Job drawing, mm, ordinate dimensions from the low corner. One solid piece. Round coordinates to 2 decimals unless told otherwise and drop trailing zeros. Loops run counter-clockwise (first coordinate to the right, second up) from the corner with the lowest first, then second, coordinate; pieces in that order, holes last.
1) Band-saw the part on D-D, the plane x = 29. Write the cut outline in (y, z) (1 decimal), then the cut area to 3 significant figures.
2) Band-saw the part on B-B, the plane x = 19.8. Write the cut outline in (y, z) (1 decimal).
3) Mould opens along Z. For the marked faces 1, 2, 3 and 4 say: +Z half, -Z half, draft (parallel to the pull), parting line (faces both ways), or undercut.
4) Drop flat-ended pins along their axis: P1, Ø2, axis at y = 1, z = 47, coming from the -X side; P2, Ø8, axis at y = 28.5, z = 35.5, coming from the +X side; P3, Ø19, axis at x = 20, y = 12.5, coming from the +Z side (1 decimal). Give the stop position or say it passes through.
5) Band-saw the part on C-C, the plane y = 15. Write the cut outline in (x, z) (1 decimal).
6) Probe line 1 (Z direction, x = 20, y = 12) (1 decimal); line 2 (Y direction, x = 19.8, z = 10.6); line 3 (Y direction, x = 16, z = 12). List the from-to ranges inside material, lowest first.
7) Band-saw the part on A-A, the plane z = 19.05. Write the cut outline in (x, y).
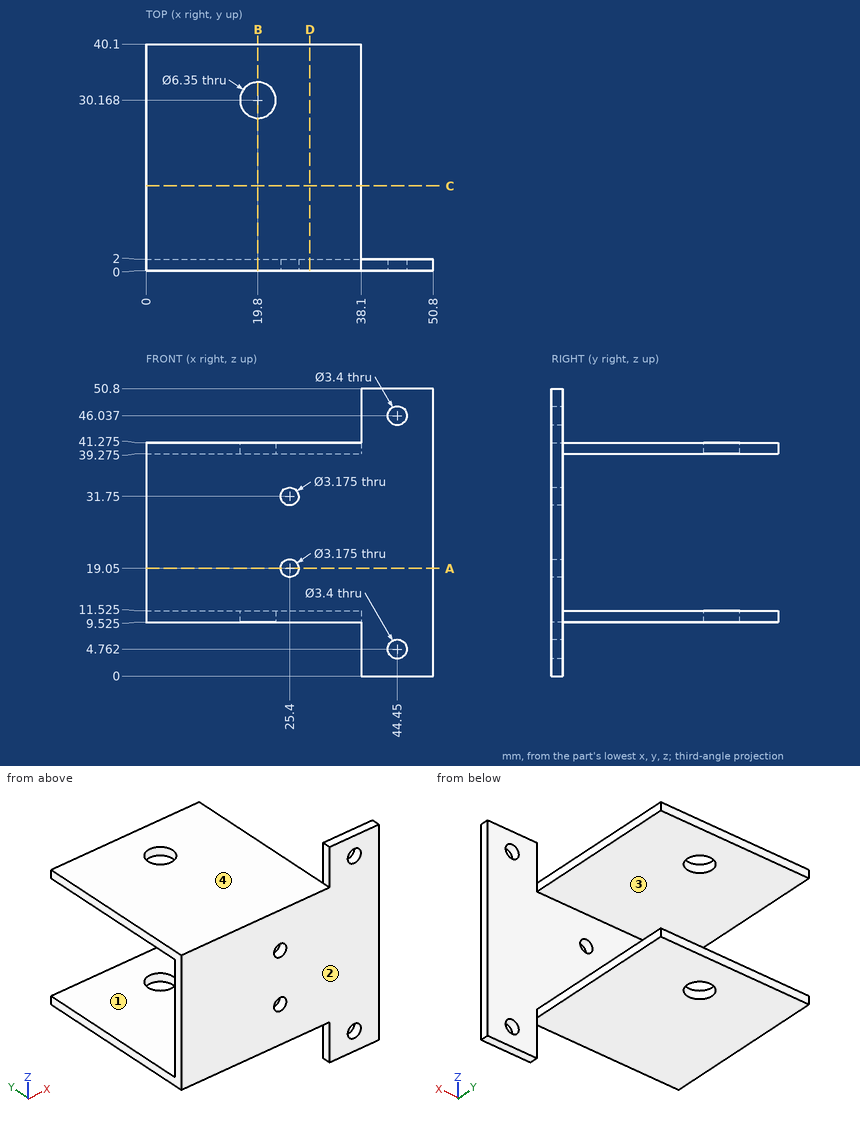
Reported:
1. outline: (0, 9.5) - (40.1, 9.5) - (40.1, 11.5) - (2, 11.5) - (2, 39.3) - (40.1, 39.3) - (40.1, 41.3) - (0, 41.3) - close
1. area: 216 mm2
2. outline: (0, 9.5) - (27, 9.5) - (27, 11.5) - (2, 11.5) - (2, 39.3) - (27, 39.3) - (27, 41.3) - (0, 41.3) - close; (33.3, 9.5) - (40.1, 9.5) - (40.1, 11.5) - (33.3, 11.5) - close; (33.3, 39.3) - (40.1, 39.3) - (40.1, 41.3) - (33.3, 41.3) - close
3. face 1: undercut
3. face 2: draft
3. face 3: undercut
3. face 4: +Z half
4. P1: stops at x = 38.1
4. P2: stops at x = 38.1
4. P3: stops at z = 41.3
5. outline: (0, 9.5) - (38.1, 9.5) - (38.1, 11.5) - (0, 11.5) - close; (0, 39.3) - (38.1, 39.3) - (38.1, 41.3) - (0, 41.3) - close
6. line 1: z = 9.5 to 11.5, 39.3 to 41.3
6. line 2: y = 0 to 26.99, 33.34 to 40.1
6. line 3: y = 0 to 2
7. outline: (0, 0) - (23.81, 0) - (23.81, 2) - (0, 2) - close; (26.99, 0) - (50.8, 0) - (50.8, 2) - (26.99, 2) - close
